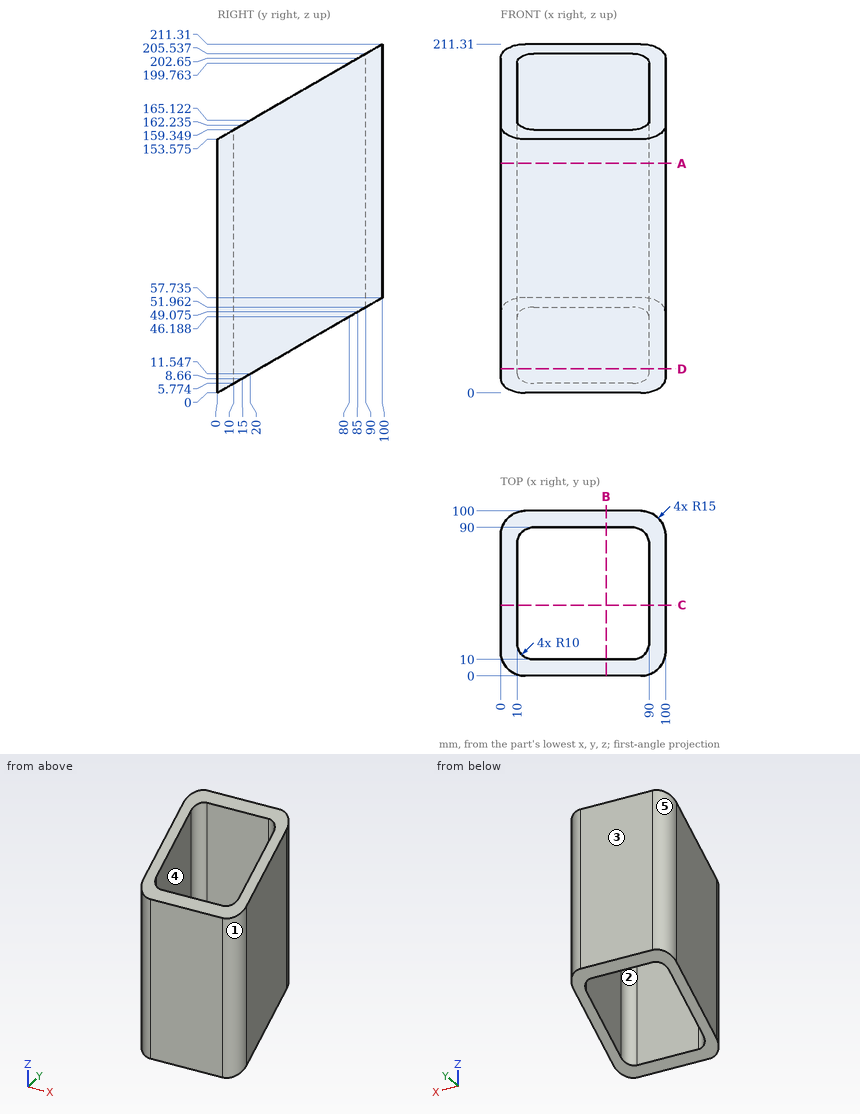
Can you work these out from the drawing? Everything is in mm from the part's minimum corner. A direction names the side the tool comes from. Coordinates: 2 decimals unless noted, no trailing zeros. Write each loop counter-clockwise with the first axis right and the second up, starting at its lowest first coordinate (ties: lowest second). Pieces come first, ordered by that corner, then holes. Notation, with made-up numbers: (1, 29) -> (24, 29) arc R27 ccw to (24, 46) -> close; hole circle Ø5 at (80, -2.5). An arc over 180 degrees is marked (long way). Write each question's results on one line, items separated by ' | '. Start each with the question number.
Item 1: On a 3-axis mill with a long thin cutter (end or side, diameter ignored), from which of +Z, -Z, +X, -X, +Y, -Y can I reach the whole of each face in a straight line? I mean the marked faces 4 and 5. Say none if no direction works.
Item 2: If we section it at B-B, the plane x = 64: Write out the boundary of the cut face in (y, z) (1 decimal), and give its area (3 significant figures).
Item 3: I'm going to push flat-ended pins straight in: P1, Ø4, axis at x = 41.5, y = 89, coming from the -Z side; P2, Ø10, axis at x = 34.5, y = 80.5, coming from the +Z side; P3, Ø4, axis at x = 11, z = 152, coming from the -Y side. Where does each tip first touch, or does it pass through?
Item 4: Please list where these lines run through material, in increasing order: probe 1 along X at (y, z) = (60.5, 123.5); probe 2 along X at (y, z) = (81, 173).
Item 5: Thinking about a two-plate mould opening in X: for the marked faces 1, 2 and 3, which applies, released by +X, released by -X, zero draft, split by the parting line, or undercut?
Item 6: If we section it at A-A, the plane z = 139: Write out the boundary of the cut face in (x, y).
Item 7: If we section it at C-C, the plane y = 43: Write out the boundary of the cut face in (x, z).
Item 8: If we section it at D-D, the plane z = 14.5: Write out the boundary of the cut face in (x, y) (1 decimal), and give its area (3 significant figures).
Answer block:
1) face 4: +Z, -Z | face 5: +Z, -Z, -X, +Y
2) outline: (0, 0) -> (10, 5.8) -> (10, 159.3) -> (0, 153.6) -> close; (90, 52) -> (100, 57.7) -> (100, 211.3) -> (90, 205.5) -> close | area: 3,070 mm²
3) P1: z = 51.96 | P2: through | P3: y = 0.13
4) probe 1: 0 to 10, 90 to 100 | probe 2: 0 to 10.05, 89.95 to 100
5) face 1: released by +X | face 2: undercut | face 3: zero draft
6) outline: (0, 15) arc R15 ccw to (15, 0) -> (85, 0) arc R15 ccw to (100, 15) -> (100, 85) arc R15 ccw to (85, 100) -> (15, 100) arc R15 ccw to (0, 85) -> close; hole (10, 20) arc R10 ccw to (20, 10) -> (80, 10) arc R10 ccw to (90, 20) -> (90, 80) arc R10 ccw to (80, 90) -> (20, 90) arc R10 ccw to (10, 80) -> close
7) outline: (0, 24.83) -> (10, 24.83) -> (10, 178.4) -> (0, 178.4) -> close; (90, 24.83) -> (100, 24.83) -> (100, 178.4) -> (90, 178.4) -> close
8) outline: (0, 15) arc R15 ccw to (15, 0) -> (85, 0) arc R15 ccw to (100, 15) -> (100, 25.1) -> (90, 25.1) -> (90, 20) arc R10 cw to (80, 10) -> (20, 10) arc R10 cw to (10, 20) -> (10, 25.1) -> (0, 25.1) -> close | area: 1,250 mm²
